Design review of the part shown in the three views and the two pictorial views. Dimensions are in mm from the part's minimum x, y and z. Round coordinates to 2 decimals unless told otherwise and drop trailing zeros. Write each loop counter-clockwise with the first axis right and the second up, starting at its lowest first coordinate (ties: lowest second). Pieces come first, ordered by that corner, then holes. Notation, with made-up numbers: (-37.5, 69.5) -> (-5.5, 69.5) arc R14 ccw to (-5.5, 76.5) -> close; hole circle Ø5 at (56, 57). An arc over 180 degrees is marked (long way). Answer as a JSON object with one key per item and string values. Group by question number.
1) We need section D-D, the plane x = 5.3. Write out the cut boundary in (y, z).
2) Insertion check: pin 1 Ø1.2 at (x, z) = (4.5, 34.5) entering from -Y; pin 2 Ø3 at (y, z) = (34, 3) entering from -X; pin 3 Ø1.2 at (x, y) = (4.5, 22) entering from -Z; pin 4 Ø12 at (y, z) = (20, 5) entering from +X. Each pin has a flat end and moves straight along its axis. Give the tip position at first contact, or say it passes through.
3) To check wall thickness, follow probe 1 along Z at (x, y) = (1.6, 34); probe 2 along Z at (x, y) = (4.9, 17); probe 3 along X at (y, z) = (20.5, 32). State the ranges of each line that lie inside material, in increasing order. Write a range as [from, to].
4) We need section B-B, the plane y = 3. Write out the cut boundary in (x, z), then the cut area to 3 significant figures.
5) We need section C-C, the plane y = 13. Write out the cut boundary in (x, z), then the cut area to 3 significant figures.
6) We need section A-A, the plane z = 3. Write out the cut boundary in (x, y), then the cut area to 3 significant figures.
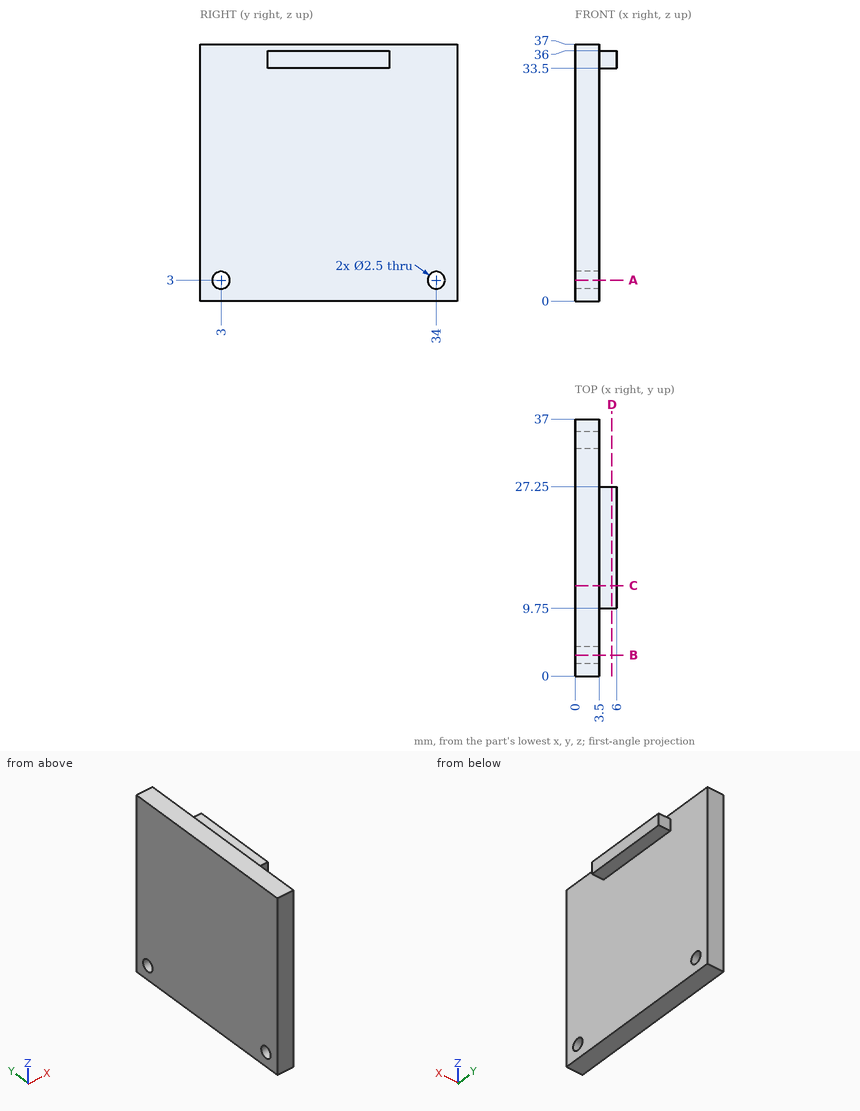
Here are the results:
{
 "1": {"outline": "(9.75, 33.5) -> (27.25, 33.5) -> (27.25, 36) -> (9.75, 36) -> close"},
 "2": {"pin 1": "stops at y = 9.75", "pin 2": "stops at x = 0", "pin 3": "stops at z = 33.5", "pin 4": "stops at x = 3.5"},
 "3": {"probe 1": "z = [0, 1.75], [4.25, 37]", "probe 2": "z = [33.5, 36]", "probe 3": "x = [0, 3.5]"},
 "4": {"outline": "(0, 0) -> (3.5, 0) -> (3.5, 1.75) -> (0, 1.75) -> close; (0, 4.25) -> (3.5, 4.25) -> (3.5, 37) -> (0, 37) -> close", "area": "121 mm^2"},
 "5": {"outline": "(0, 0) -> (3.5, 0) -> (3.5, 33.5) -> (6, 33.5) -> (6, 36) -> (3.5, 36) -> (3.5, 37) -> (0, 37) -> close", "area": "136 mm^2"},
 "6": {"outline": "(0, 0) -> (3.5, 0) -> (3.5, 1.75) -> (0, 1.75) -> close; (0, 4.25) -> (3.5, 4.25) -> (3.5, 32.75) -> (0, 32.75) -> close; (0, 35.25) -> (3.5, 35.25) -> (3.5, 37) -> (0, 37) -> close", "area": "112 mm^2"}
}
